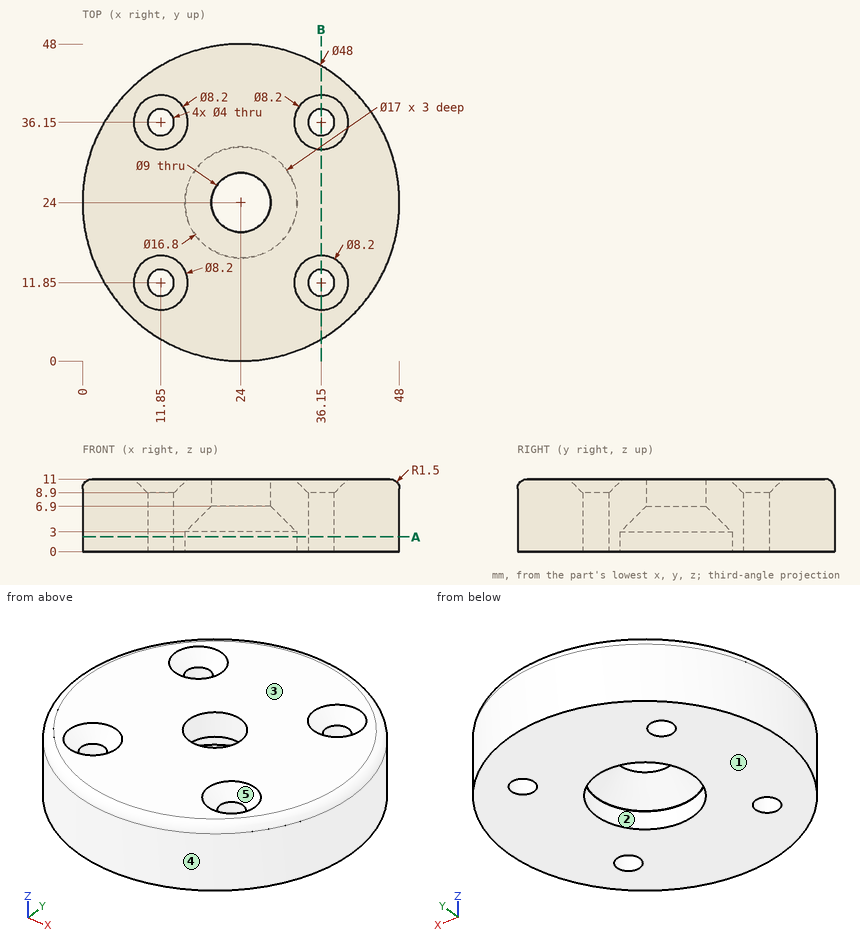
Geometry: see drawing. Coordinates: mm, zero at the bounding-box minimum. A direction names the side the tool comes from. Coordinates: 2 decimals unless noted, no trailing zeros. Write each loop counter-clockwise with the first axis right and the second up, starting at its lowest first coordinate (ties: lowest second). Pieces come first, ordered by that corner, then holes.
1) Material intervals for line 1 along Y through (x, z) = (35, 3); line 2 along Y through (x, z) = (36.15, 7); line 3 along X through (y, z) = (35.5, 3), sorted ascending.
2) Pin query (flat end, axial travel): pin 1 Ø4 at (y, z) = (34.5, 3.5) entering from -X; pin 2 Ø11.5 at (x, y) = (24, 24) entering from -Z; pin 3 Ø2 at (x, z) = (28.5, 5.5) entering from -Y. Return the tip coordinate at first contact, or that it passes through.
3) Set-up query: the marked faces 1 and 2. Return all of +Z, -Z, +X, -X, +Y, -Y with unobstructed straight access to the full face (end or side cutting, diameter ignored); none if empty.
4) Section B-B on x = 36.15. State how many separate pieces and enclosed holes the cut face has, and give its area (3 significant figures).
5) Mould query, pull axis X, two halves, no side actions, for the marked faces 3, 4 and 5. Classes: pulls with the +X half, pulls with the -X half, needs draft (parallel to the pull), parting line crosses it, or undercut.
6) Section A-A on z = 2.25. Output: boundary loops of the cut face in (x, y), and give its area (3 significant figures).
Check result:
1. line 1: y = 2.67 to 10.21, 13.49 to 34.51, 37.79 to 45.33
1. line 2: y = 3.3 to 9.85, 13.85 to 34.15, 38.15 to 44.7
1. line 3: x = 2.93 to 9.96, 13.74 to 34.26, 38.04 to 45.07
2. pin 1: stops at x = 1.56
2. pin 2: stops at z = 5.65
2. pin 3: stops at y = 0.26
3. face 1: -Z, +X, -X, +Y, -Y
3. face 2: -Z
4. separate pieces: 3
4. enclosed holes: 0
4. area: 357 mm2
5. face 3: needs draft
5. face 4: parting line crosses it
5. face 5: undercut
6. outline: circle Ø48 at (24, 24); hole circle Ø4 at (11.85, 11.85); hole circle Ø4 at (11.85, 36.15); hole circle Ø17 at (24, 24); hole circle Ø4 at (36.15, 11.85); hole circle Ø4 at (36.15, 36.15)
6. area: 1,530 mm2
